Source: CAD feature listing. Evaluate the final solid. Frame: model axes, mm. A direction names the side the tool comes from. Give positions to 0.01 mm unless a question says otherwise; leave off trailing zeros. Order: outer loops, then holes, each group sorted by start corner. A loop starts at its lowest first (then second) coordinate and runs counter-clockwise, first axis right, second up.
1) Access query for faces 4 (the face through (-20.405, 2, -32)), 5 (the face through (-72, 6.096, -30)), 6 (the face through (-26.247, 5, -26)). Directions: +Z, -Z, +X, -X, +Y, -Y. A direction counts if a zero-diameter tool reaches every point of the face in a straight line with its end or side. Return the directions, or none.
2) First-contact query: P1, Ø1.3, axis at y = 3, z = -32, coming from the +X side; P2, Ø1.4, axis at y = -1, z = -27, coming from the -X side; P3, Ø6, axis at x = -20.4, z = -25.89, coming from the +Y side. Flat tips, straight axial feed; report the tip coordinate or a pass-through.
3) Draft query along Z for faces 1 (the face through (-59, 0, -33)), 2 (the face through (-74.01, 6.58, -28.47)), 3 (the face through (-69, 3, -16.839)). Return one class per face: released by +Z, released by -Z, zero draft, split by the parting line, or undercut.
4) Section D-D, the plane x = -91. Return loops of the section in (y, z).
5) Section C-C, the plane z = -31. Return loops of the section in (x, y), plus the area to 3 significant figures.
6) Material intervals for line 1 (Y direction, x = -50, z = -29.75); line 2 (X direction, y = 5, z = -32.5); line 3 (X direction, y = 2.25, z = -32.5), sorted ascending.
7) Section B-B, the plane y = 2. Return loops of the section in (x, z) (1 decimal).
8) Section A-A, the plane x = -101. Return loops of the section in (y, z), plus the area to 3 significant figures.
```python
from build123d import *

# Parameters (mm, degrees)
SKETCH1_W           = 99.568
SKETCH1_H           = 18.1102
BOSS_EXTRUDE1_DEPTH = 6.096
SKETCH2_W           = 9.652
SKETCH2_H           = 18.1102
CUT_EXTRUDE1_DEPTH  = 1.778
SKETCH3_R           = 1.905
CUT_EXTRUDE2_DEPTH  = 5.318
SKETCH4_R           = 3.937
CUT_EXTRUDE3_DEPTH  = 1.27
SKETCH5_W           = 82.55
SKETCH5_H           = 12.7
BOSS_EXTRUDE2_DEPTH = 1.27
CUT_EXTRUDE4_DEPTH  = 6.588
SKETCH8_R           = 3.81
BOSS_EXTRUDE3_DEPTH = 3.556


with BuildPart() as part:
    # Sketch1 → Boss-Extrude1 (new body)
    with BuildSketch(Plane(origin=(0, 0, 0), x_dir=(1, 0, 0), z_dir=(0, 1, 0))):
        with Locations((-66.378666667, 25.894273737)):
            Rectangle(SKETCH1_W, SKETCH1_H)
    extrude(amount=BOSS_EXTRUDE1_DEPTH)

    # Sketch2 → Cut-Extrude1 (cut)
    with BuildSketch(Plane(origin=(0, 6.096, 0), x_dir=(1, 0, 0), z_dir=(0, 1, 0))):
        with Locations((-21.420666667, 25.894273737)):
            Rectangle(SKETCH2_W, SKETCH2_H)
    extrude(amount=-CUT_EXTRUDE1_DEPTH, mode=Mode.SUBTRACT)

    # Sketch3 → Cut-Extrude2 (cut, through all)
    with BuildSketch(Plane(origin=(0, 4.318, 0), x_dir=(1, 0, 0), z_dir=(0, 1, 0))):
        with Locations((-20.404666667, 25.894273737)):
            Circle(SKETCH3_R)
    extrude(amount=-CUT_EXTRUDE2_DEPTH, mode=Mode.SUBTRACT)

    # Sketch4 → Cut-Extrude3 (cut)
    with BuildSketch(Plane(origin=(0, 6.096, 0), x_dir=(1, 0, 0), z_dir=(0, 1, 0))):
        with Locations((-33.104666667, 25.894273737)):
            Circle(SKETCH4_R)
        with Locations((-52.154666667, 25.894273737)):
            Circle(SKETCH4_R)
        with Locations((-71.204666667, 25.894273737)):
            Circle(SKETCH4_R)
        with Locations((-90.254666667, 25.894273737)):
            Circle(SKETCH4_R)
        with Locations((-109.304666667, 25.894273737)):
            Circle(SKETCH4_R)
    extrude(amount=-CUT_EXTRUDE3_DEPTH, mode=Mode.SUBTRACT)

    # Sketch5 → Boss-Extrude2 (add)
    with BuildSketch(Plane.XZ):
        with Locations((-71.204666667, -25.894273737)):
            Rectangle(SKETCH5_W, SKETCH5_H)
    extrude(amount=BOSS_EXTRUDE2_DEPTH)

    # Sketch7 → Cut-Extrude4 (cut, through all)
    with BuildSketch(Plane(origin=(0, 4.318, 0), x_dir=(1, 0, 0), z_dir=(0, 1, 0))):
        with BuildLine():
            Line((-16.594666667, 34.949373737), (-20.404666667, 34.949373737))
            Line((-20.404666667, 34.949373737), (-20.404666667, 29.680045052))
            ThreePointArc((-20.404666667, 29.680045052), (-16.618895352, 25.894273737), (-20.404666667, 22.108502422))
            Line((-20.404666667, 22.108502422), (-20.404666667, 16.839173737))
            Line((-20.404666667, 16.839173737), (-16.594666667, 16.839173737))
            Line((-16.594666667, 16.839173737), (-16.594666667, 34.949373737))
        make_face()
    extrude(amount=-CUT_EXTRUDE4_DEPTH, mode=Mode.SUBTRACT)

    # Sketch8 → Boss-Extrude3 (add)
    with BuildSketch(Plane(origin=(0, 4.826, 0), x_dir=(1, 0, 0), z_dir=(0, 1, 0))):
        with Locations((-33.104666667, 25.894273737)):
            Circle(SKETCH8_R)
        with Locations((-52.154666667, 25.894273737)):
            Circle(SKETCH8_R)
        with Locations((-71.204666667, 25.894273737)):
            Circle(SKETCH8_R)
        with Locations((-90.254666667, 25.894273737)):
            Circle(SKETCH8_R)
        with Locations((-109.304666667, 25.894273737)):
            Circle(SKETCH8_R)
    extrude(amount=BOSS_EXTRUDE3_DEPTH)


solid = part.part
```
From the geometry:
1. face 4: -Z, +X, +Y, -Y
1. face 5: +Y
1. face 6: +Z, -Z, +X, +Y
2. P1: stops at x = -20.4
2. P2: stops at x = -112.48
2. P3: stops at y = 4.32
3. face 1: zero draft
3. face 2: undercut
3. face 3: released by +Z
4. outline: (-1.27, -32.24) - (0, -32.24) - (0, -34.95) - (6.1, -34.95) - (6.1, -29.76) - (4.83, -29.76) - (4.83, -29.63) - (8.38, -29.63) - (8.38, -22.16) - (4.83, -22.16) - (4.83, -22.03) - (6.1, -22.03) - (6.1, -16.84) - (0, -16.84) - (0, -19.54) - (-1.27, -19.54) - close
5. outline: (-116.16, 0) - (-112.48, 0) - (-112.48, -1.27) - (-29.93, -1.27) - (-29.93, 0) - (-20.4, 0) - (-20.4, 4.32) - (-26.25, 4.32) - (-26.25, 6.1) - (-116.16, 6.1) - close
5. area: 678 mm2
6. line 1: y = -1.27 to 6.1
6. line 2: x = -116.16 to -26.25
6. line 3: x = -116.16 to -20.4
7. outline: (-116.2, -34.9) - (-20.4, -34.9) - (-20.4, -29.7) arc R3.8 ccw to (-20.4, -22.1) - (-20.4, -16.8) - (-116.2, -16.8) - close; hole circle Ø3.8 at (-20.4, -25.9)
8. outline: (-1.27, -32.24) - (0, -32.24) - (0, -34.95) - (6.1, -34.95) - (6.1, -16.84) - (0, -16.84) - (0, -19.54) - (-1.27, -19.54) - close
8. area: 127 mm2
